Source: CAD feature listing. Evaluate the final solid. Frame: model axes, mm. A direction names the side the tool comes from. Round coordinates to 2 decimals unless told otherwise and drop trailing zeros. Order: outer loops, then holes, each group sorted by start corner. A loop starts at its lowest first (then second) coordinate and runs counter-clockwise, first axis right, second up. Notation, with made-up numbers: (48, 33.5) -> (68, 33.5) arc R29 ccw to (68, 59.5) -> close; hole circle Ø4 at (70.25, 58.5). An arc over 180 degrees is marked (long way). Write item = value, one per line. Start each with the question number.
(1) Reachability of faces 1 (the face through (33, -9, 38.1)), 2 (the face through (110.19, -9.39, -232.51)), 3 (the face through (-111.998, -9.392, -124.339)), 4 (the face through (132.19, -9.39, -195.19)) from +Z, -Z, +X, -X, +Y, -Y: full face, straight path, thin tool, end or side. Return the list, or none.
(2) Cut plane A-A on z = 215.9. Return the cut outline in (x, y), then the cut area to 3 significant figures.
(3) Cut plane C-C on y = -12.5. Give the number of separate pieces and of enclosed holes in the cut face, then the cut area to 3 significant figures.
(4) Draft query along X for faces 5 (the face through (12.7, -9, -39)), 6 (the face through (-171.591, -9.392, -83.016)), 7 (the face through (37, -19.05, -50)). Return one class per face: released by +X, released by -X, zero draft, split by the parting line, or undercut.
(5) Contact query for flat-ended pins moving along their axis: pin 1 Ø2 at (x, y) = (-112.5, -10) entering from +Z; pin 2 Ø4 at (y, z) = (-7, 30.5) entering from +X; pin 3 Ø10 at (x, y) = (-49, -6) entering from -Z. Output: stop coordinate, or through.
(6) Ray query, line 1 (Z direction, x = 127, y = -11.5); line 2 (Z direction, x = 118.5, y = -12); line 3 (X direction, y = -2.25, z = 204). Return the intervals inside material, ascending.
(7) Cut plane B-B on x = -49. Return the cut outline in (y, z), then the cut area to 3 significant figures.
from build123d import *

# Parameters (mm, degrees)
F0_R     = 4.953
F0_R_2   = 3.175
F0_R_3   = 5.1562
F0_R_4   = 3.96875
F1_DEPTH = 19.05


# Not quite as in the source:
# - ends of sketch curves that miss each other by under 0.0002 mm in the source are joined


with BuildPart() as f1:
    # F0 (on Front) → F1 (new body)
    with BuildSketch(Plane.XZ):
        with BuildLine():
            ThreePointArc((177.8, 25.4), (174.0802561211, 34.3802561211), (165.1, 38.1))
            Line((165.1, 38.1), (150.8125, 38.1))
            ThreePointArc((150.8125, 38.1), (142.6824039546, 34.7324039546), (146.05, 42.8625))
            Line((146.05, 42.8625), (146.05, 228.6))
            ThreePointArc((146.05, 228.6), (142.3302561211, 237.5802561211), (133.35, 241.3))
            Line((133.35, 241.3), (57.15, 241.3))
            ThreePointArc((57.15, 241.3), (48.1697438789, 237.5802561211), (44.45, 228.6))
            Line((44.45, 228.6), (44.45, 42.8625))
            ThreePointArc((44.45, 42.8625), (47.8175960454, 34.7324039546), (39.6875, 38.1))
            Line((39.6875, 38.1), (25.4, 38.1))
            ThreePointArc((25.4, 38.1), (16.4197438789, 34.3802561211), (12.7, 25.4))
            Line((12.7, 25.4), (12.7, -104.775))
            ThreePointArc((12.7, -104.775), (6.1904482119, -120.4904482119), (-9.525, -127))
            Line((-9.525, -127), (-101.4522228, -127))
            ThreePointArc((-101.4522228, -127), (-112.1350976667, -124.2641459429), (-120.1878905046, -116.7301403448))
            Line((-120.1878905046, -116.7301403448), (-139.4968508, -86.469855))
            ThreePointArc((-139.4968508, -86.469855), (-146.9715660509, -79.2640655101), (-156.9037505938, -76.2397575751))
            ThreePointArc((-156.9037505938, -76.2397575751), (-171.7534129546, -83.1865755647), (-177.8, -98.425))
            Line((-177.8, -98.425), (-177.8, -219.075))
            ThreePointArc((-177.8, -219.075), (-171.2904482119, -234.7904482119), (-155.575, -241.3))
            Line((-155.575, -241.3), (-128.5875, -241.3))
            Line((-128.5875, -241.3), (-98.5712024, -223.970088))
            Line((-98.5712024, -223.970088), (95.3962024, -223.970088))
            Line((95.3962024, -223.970088), (125.4125, -241.3))
            Line((125.4125, -241.3), (155.575, -241.3))
            ThreePointArc((155.575, -241.3), (171.2904482119, -234.7904482119), (177.8, -219.075))
            Line((177.8, -219.075), (177.8, 25.4))
        make_face()
        with BuildLine():
            Line((-137.639425, -205.5625302), (-143.989425, -194.564))
            ThreePointArc((-143.989425, -194.564), (-142.1764994912, -187.7980758813), (-135.4105758813, -189.6110005088))
            Line((-135.4105758813, -189.6110005088), (-129.060575, -200.6095302))
            ThreePointArc((-129.060575, -200.6095302), (-128.4232829137, -202.5764541494), (-128.6445091035, -204.6321752201))
            Line((-128.6445091035, -204.6321752201), (-126.1204742, -209.0039))
            ThreePointArc((-126.1204742, -209.0039), (-124.4219046114, -218.5499378494), (-131.8397164566, -212.3058998322))
            Line((-131.8397164566, -212.3058998322), (-134.3637394, -207.934179))
            ThreePointArc((-134.3637394, -207.934179), (-136.2546626338, -207.0979055699), (-137.639425, -205.5625302))
        make_face(mode=Mode.SUBTRACT)
        with Locations((-155.575, -98.425)):
            Circle(F0_R, mode=Mode.SUBTRACT)
        with Locations((34.925, -164.051488)):
            Circle(F0_R_2, mode=Mode.SUBTRACT)
        with Locations((34.925, -129.126488)):
            Circle(F0_R_2, mode=Mode.SUBTRACT)
        with BuildLine():
            Line((129.060575, -200.6095302), (135.410575, -189.611))
            ThreePointArc((135.410575, -189.611), (142.1764994912, -187.7980758813), (143.9894241187, -194.5639994912))
            Line((143.9894241187, -194.5639994912), (137.639425, -205.5625302))
            ThreePointArc((137.639425, -205.5625302), (136.2546626338, -207.0979055699), (134.3637392893, -207.9341784706))
            Line((134.3637392893, -207.9341784706), (131.839716, -212.3059))
            ThreePointArc((131.839716, -212.3059), (124.4219046114, -218.5499378494), (126.1204745175, -209.0039018342))
            Line((126.1204745175, -209.0039018342), (128.6444976, -204.632179))
            ThreePointArc((128.6444976, -204.632179), (128.4232829137, -202.5764541494), (129.060575, -200.6095302))
        make_face(mode=Mode.SUBTRACT)
        with Locations((34.925, -38.1)):
            Circle(F0_R_2, mode=Mode.SUBTRACT)
        with Locations((149.225, -98.425)):
            Circle(F0_R, mode=Mode.SUBTRACT)
        with Locations((155.575, -38.1)):
            Circle(F0_R_2, mode=Mode.SUBTRACT)
        with Locations((34.925, 12.7)):
            Circle(F0_R_2, mode=Mode.SUBTRACT)
        with Locations((60.325, 63.5)):
            Circle(F0_R_3, mode=Mode.SUBTRACT)
        with Locations((73.025, 101.6)):
            Circle(F0_R_4, mode=Mode.SUBTRACT)
        with Locations((155.575, 12.7)):
            Circle(F0_R_2, mode=Mode.SUBTRACT)
        with Locations((130.175, 63.5)):
            Circle(F0_R_3, mode=Mode.SUBTRACT)
        with Locations((117.475, 101.6)):
            Circle(F0_R_4, mode=Mode.SUBTRACT)
        with Locations((60.325, 139.7)):
            Circle(F0_R_3, mode=Mode.SUBTRACT)
        with Locations((73.025, 177.8)):
            Circle(F0_R_4, mode=Mode.SUBTRACT)
        with Locations((60.325, 215.9)):
            Circle(F0_R_3, mode=Mode.SUBTRACT)
        with Locations((130.175, 139.7)):
            Circle(F0_R_3, mode=Mode.SUBTRACT)
        with Locations((117.475, 177.8)):
            Circle(F0_R_4, mode=Mode.SUBTRACT)
        with Locations((95.25, 231.775)):
            Circle(F0_R_2, mode=Mode.SUBTRACT)
        with Locations((130.175, 215.9)):
            Circle(F0_R_3, mode=Mode.SUBTRACT)
    extrude(amount=F1_DEPTH)


solid = f1.part
Evaluation:
q1.face_1 = +Z, -X, +Y, -Y
q1.face_2 = -Z, +Y, -Y
q1.face_3 = +Z, +Y, -Y
q1.face_4 = +Y, -Y
q2.outline = (44.45, -19.05) -> (55.17, -19.05) -> (55.17, 0) -> (44.45, 0) -> close; (65.48, -19.05) -> (125.02, -19.05) -> (125.02, 0) -> (65.48, 0) -> close; (135.33, -19.05) -> (146.05, -19.05) -> (146.05, 0) -> (135.33, 0) -> close
q2.area = 1,540 mm^2
q3.separate_pieces = 1
q3.enclosed_holes = 21
q3.area = 85,000 mm^2
q4.face_5 = undercut
q4.face_6 = released by -X
q4.face_7 = zero draft
q5.pin_1 = -123.45
q5.pin_2 = 177.42
q5.pin_3 = -223.97
q6.line_1 = -241.3 to -219.24, -207.48 to 59.44, 67.56 to 135.64, 143.76 to 211.84, 219.96 to 241.3
q6.line_2 = -237.31 to 97.77, 105.43 to 173.97, 181.63 to 241.3
q6.line_3 = 44.45 to 146.05
q7.outline = (-19.05, -223.97) -> (0, -223.97) -> (0, -127) -> (-19.05, -127) -> close
q7.area = 1,850 mm^2
